from build123d import *

# Parameters (mm, degrees)
SKETCH1_R           = 75
BOSS_EXTRUDE1_DEPTH = 3.175
CUT_EXTRUDE1_DEPTH  = 3.175
SKETCH3_R           = 1.778
SKETCH3_R_2         = 1.5875
CUT_EXTRUDE2_DEPTH  = 3.175
SKETCH4_R           = 1.5875
CUT_EXTRUDE3_DEPTH  = 3.175
CUT_EXTRUDE4_DEPTH  = 3.175


with BuildPart() as part:
    # Sketch1 → Boss-Extrude1 (new body)
    with BuildSketch(Plane(origin=(0, 0, 0), x_dir=(1, 0, 0), z_dir=(0, 1, 0))):
        Circle(SKETCH1_R)
    extrude(amount=BOSS_EXTRUDE1_DEPTH)

    # Sketch2 → Cut-Extrude1 (cut)
    with BuildSketch(Plane(origin=(0, 3.175, 0), x_dir=(1, 0, 0), z_dir=(0, 1, 0))):
        with BuildLine():
            Line((-56.262005909, -49.594220339), (56.262005909, -49.594220339))
            ThreePointArc((56.262005909, -49.594220339), (0, -75), (-56.262005909, -49.594220339))
        make_face()
        with BuildLine():
            Line((-56.262005909, 49.594220339), (56.262005909, 49.594220339))
            ThreePointArc((56.262005909, 49.594220339), (0, 75), (-56.262005909, 49.594220339))
        make_face()
    extrude(amount=-CUT_EXTRUDE1_DEPTH, mode=Mode.SUBTRACT)

    # Sketch3 → Cut-Extrude2 (cut)
    with BuildSketch(Plane(origin=(0, 3.175, 0), x_dir=(1, 0, 0), z_dir=(0, 1, 0))):
        with Locations((0, 36.894220339)):
            Circle(SKETCH3_R)
        with Locations((0, 11.494220339)):
            Circle(SKETCH3_R)
        with Locations((0, 17.844220339)):
            Circle(SKETCH3_R)
        with Locations((0, 24.194220339)):
            Circle(SKETCH3_R)
        with Locations((0, 30.544220339)):
            Circle(SKETCH3_R)
        with Locations((0, -11.494220339)):
            Circle(SKETCH3_R)
        with Locations((0, -17.844220339)):
            Circle(SKETCH3_R)
        with Locations((0, -24.194220339)):
            Circle(SKETCH3_R)
        with Locations((0, -30.544220339)):
            Circle(SKETCH3_R)
        with Locations((0, -36.894220339)):
            Circle(SKETCH3_R)
        with Locations((-52.180304588, -44.729838125)):
            Circle(SKETCH3_R_2)
        with Locations((52.180304588, -44.729838125)):
            Circle(SKETCH3_R_2)
        with Locations((52.180304588, 44.729838125)):
            Circle(SKETCH3_R_2)
        with Locations((-52.180304588, 44.729838125)):
            Circle(SKETCH3_R_2)
        with Locations((-19.05, 44.729838125)):
            Circle(SKETCH3_R_2)
        with Locations((-19.05, -44.729838125)):
            Circle(SKETCH3_R_2)
        with Locations((19.05, -44.729838125)):
            Circle(SKETCH3_R_2)
        with Locations((19.05, 44.729838125)):
            Circle(SKETCH3_R_2)
    extrude(amount=-CUT_EXTRUDE2_DEPTH, mode=Mode.SUBTRACT)

    # Sketch4 → Cut-Extrude3 (cut)
    with BuildSketch(Plane(origin=(0, 3.175, 0), x_dir=(1, 0, 0), z_dir=(0, 1, 0))):
        with Locations((-60.791780161, 34.29)):
            Circle(SKETCH4_R)
        with Locations((-17.611780161, 34.29)):
            Circle(SKETCH4_R)
        with Locations((-17.611780161, -34.29)):
            Circle(SKETCH4_R)
        with Locations((-60.791780161, -34.29)):
            Circle(SKETCH4_R)
    cut_extrude3 = extrude(amount=-CUT_EXTRUDE3_DEPTH, mode=Mode.SUBTRACT)

    # Sketch5 → Cut-Extrude4 (cut)
    with BuildSketch(Plane(origin=(0, 3.175, 0), x_dir=(1, 0, 0), z_dir=(0, 1, 0))):
        with BuildLine():
            Line((-68.527144986, 30.48), (-21.421780161, 30.48))
            Line((-21.421780161, 30.48), (-21.421780161, -30.48))
            Line((-21.421780161, -30.48), (-68.527144986, -30.48))
            ThreePointArc((-68.527144986, -30.48), (-75, 0), (-68.527144986, 30.48))
        make_face()
    cut_extrude4 = extrude(amount=-CUT_EXTRUDE4_DEPTH, mode=Mode.SUBTRACT)

    # Mirror1: Cut-Extrude3, Cut-Extrude4 across plane
    add(cut_extrude3.mirror(Plane(origin=(0, 0, 0), x_dir=(0, 0, 1), z_dir=(1, 0, 0))), mode=Mode.SUBTRACT)
    add(cut_extrude4.mirror(Plane(origin=(0, 0, 0), x_dir=(0, 0, 1), z_dir=(1, 0, 0))), mode=Mode.SUBTRACT)


solid = part.part
Build history of the part. All positions in model axes, mm. A direction names the side the tool comes from. Round coordinates to 2 decimals unless told otherwise and drop trailing zeros. Write each loop counter-clockwise with the first axis right and the second up, starting at its lowest first coordinate (ties: lowest second). Pieces come first, ordered by that corner, then holes. Notation, with made-up numbers: (48.5, 36) -> (90.5, 36) arc R13 ccw to (90.5, 40) -> close; hole circle Ø9 at (77, -15). An arc over 180 degrees is marked (long way). Use one line per item in the form item = value.
Q1. Drop flat-ended pins along their axis: P1, Ø1, axis at y = 2, z = -12.5, coming from the +X side; P2, Ø3, axis at x = 0, z = -11.49, coming from the +Y side; P3, Ø1, axis at y = 2, z = -7, coming from the -X side. Give the stop position or say it passes through.
Conclusion:
P1 = 21.42
P2 = through
P3 = -21.42
Q2. Two-plate mould, pull along X, no slides. Class faces 3 (the cylindrical face through (-0.39, 1.61, 38.63)), 4 (the flat face through (-1, 2, -49.594)): released by +X, released by -X, zero draft, split by the parting line, or undercut.
Conclusion:
face_3 = undercut
face_4 = zero draft
Q3. Drill centre lines: L1, parallel to Z at x = -47, y = 2.6; L2, parallel to Z at x = 60, y = 1.7; L3, parallel to X at y = 1.9, z = 34.29. Where is each one in solid material? Low to high.
Conclusion:
L1 = -49.59 to -30.48, 30.48 to 49.59
L2 = -45 to -35.67, -32.91 to -30.48, 30.48 to 32.91, 35.67 to 45
L3 = -66.7 to -62.38, -59.2 to -19.2, -16.02 to 16.02, 19.2 to 59.2, 62.38 to 66.7
Q4. Tool access for faces 1 (the flat face through (45, 2, 30.48)), 2 (the cylindrical face through (-18.87, 1.61, 35.26)): list every direction of +Z, -Z, +X, -X, +Y, -Y with a clear straight run to the whole face (end or side of a thin tool).
Conclusion:
face_1 = +X, +Y, -Y
face_2 = +Y, -Y
Q5. Band-saw the part on B-B, the plane y = 2. State how many separate pieces and enclosed holes the cut face has, then the cut area to 3 significant figures.
Conclusion:
separate_pieces = 1
enclosed_holes = 26
area = 7,210 mm²
Q6. Band-saw the part on A-A, the plane x = -45. Write the cut outline in (y, z) (3 decimals).
Conclusion:
outline = (0, -49.594) -> (3.175, -49.594) -> (3.175, -30.48) -> (0, -30.48) -> close; (0, 30.48) -> (3.175, 30.48) -> (3.175, 49.594) -> (0, 49.594) -> close
Q7. Band-saw the part on D-D, the plane z = -7. Write the cut outline in (x, y) (3 decimals), then the cut area to 3 significant figures.
Conclusion:
outline = (-21.422, 0) -> (21.422, 0) -> (21.422, 3.175) -> (-21.422, 3.175) -> close
area = 136 mm²
